Part model, mm, in its own coordinate system. Face numbers are marked on the shaded views. A direction names the side the tool comes from. Give positions to 0.01 mm unless a question says otherwise; leave off trailing zeros. Order: outer loops, then holes, each group sorted by start corner. A loop starts at its lowest first (then second) coordinate and runs counter-clockwise, first axis right, second up. Notation, with made-up numbers: (-15, 3.5) - (-3, 3.5) arc R18 ccw to (-3, 19.5) - close; hole circle Ø5 at (32.5, 24). An arc over 180 degrees is marked (long way). One line per item, written item: value.
```python
from build123d import *

# Parameters (mm, degrees)
F1_DEPTH = 25.4


with BuildPart() as f1:
    # F0 (on Right) → F1 (new body)
    with BuildSketch(Plane.YZ):
        with BuildLine():
            Line((-36.9195081294, 56.1760254204), (-56.0708381236, 56.1760254204))
            Line((-56.0708381236, 56.1760254204), (-56.0708381236, 0))
            Line((-56.0708381236, 0), (-16.9170089066, 0))
            add(Edge.make_bspline(
                [(-36.9195081294, 35.9607338905), (-35.4601229338, 35.3580538857), (-32.1631189369, 33.9964953399), (-25.8800850757, 28.9915492914), (-20.347271317, 19.1454647502), (-15.8846570192, 11.4601698018), (-15.6661719788, 4.0056512293), (-16.1933271118, -0.2408932737), (-16.7678721462, -0.0496434244), (-16.9170089066, 0)],
                knots=[0, 0, 0, 0, 0.1333911224, 0.3013536556, 0.5037239231, 0.6830726009, 0.8493105973, 0.9608849994, 1, 1, 1, 1], degree=3))
            Line((-36.9195081294, 35.9607338905), (-36.9195081294, 56.1760254204))
        make_face()
    extrude(amount=F1_DEPTH)


solid = f1.part
```
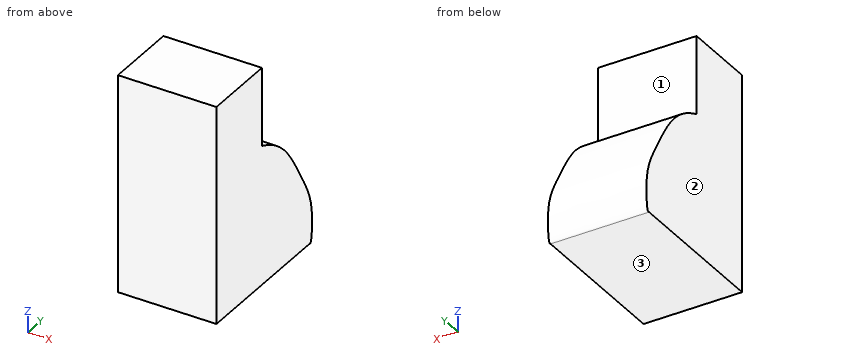
1) Pin check, flat tip, straight feed: pin 1 (8 mm diameter, centred on x = 21, y = -30.5, fed in from -Z). Stop position of the tip, or through.
Outcome:
pin 1: stops at z = 0
2) Which spindle directions (+Z, -Z, +X, -X, +Y, -Y) get a long thin tool onto all of the face, cutting with end or side? Do the marked faces 1, 2 and 3. Say none if no direction does.
Outcome:
face 1: +Z, +X, -X, +Y
face 2: +Z, -Z, -X, +Y, -Y
face 3: -Z, +X, -X, -Y
3) Cut at A-A, the plane z = 37. Give the cut face in (x, y), then the cut area to 3 significant figures.
Outcome:
outline: (0, -56.07) - (25.4, -56.07) - (25.4, -36.92) - (0, -36.92) - close
area: 486 mm^2
4) Drill centre lines: line 1 along Z through (x, y) = (7.5, -46); line 2 along Y through (x, z) = (12.25, 39); line 3 along Y through (x, z) = (14, 5). Where is each one in solid material? Low to high. Write a range as from..to.
Outcome:
line 1: z = 0..56.18
line 2: y = -56.07..-36.92
line 3: y = -56.07..-15.8
